Autodesk Inventor part; units mm, degrees
ref_plane "Plano inicial" through (0, 0, -25.4) normal (0, 0, 1) x (1, 0, 0)
ref_plane "Plano final" through (0, 0, 2215.4) normal (0, 0, 1) x (1, 0, 0)
ref_plane "Plano de trabajo4" through (0, 25.4, 2215.4) normal (0, -0.7071, 0.7071) x (1, 0, 0)
ref_plane "Plano inicial" through (0, 0, -25.4) normal (0, 0, 1) x (1, 0, 0)
ref_plane "Plano final" through (0, 0, 2215.4) normal (0, 0, 1) x (1, 0, 0)
sketch "Boceto" plane through (0, 0, 0) normal (0, 0, 1) x (1, 0, 0)
  line L0 (-25.4, -19.05) -> (-25.4, 19.05)
  line L1 (-19.05, 25.4) -> (19.05, 25.4)
  line L2 (25.4, 19.05) -> (25.4, -19.05)
  line L3 (19.05, -25.4) -> (-19.05, -25.4)
  arc A0 (-25.4, -19.05) -> (-19.05, -25.4) centre (-19.05, -19.05) ccw
  arc A1 (-19.05, 25.4) -> (-25.4, 19.05) centre (-19.05, 19.05) ccw
  arc A2 (25.4, 19.05) -> (19.05, 25.4) centre (19.05, 19.05) ccw
  arc A3 (19.05, -25.4) -> (25.4, -19.05) centre (19.05, -19.05) ccw
  arc A4 (-19.05, 22.225) -> (-22.225, 19.05) centre (-19.05, 19.05) ccw
  line L4 (-19.05, 22.225) -> (19.05, 22.225)
  arc A5 (22.225, 19.05) -> (19.05, 22.225) centre (19.05, 19.05) ccw
  line L5 (22.225, 19.05) -> (22.225, -19.05)
  arc A6 (19.05, -22.225) -> (22.225, -19.05) centre (19.05, -19.05) ccw
  line L6 (19.05, -22.225) -> (-19.05, -22.225)
  arc A7 (-22.225, -19.05) -> (-19.05, -22.225) centre (-19.05, -19.05) ccw
  line L7 (-22.225, -19.05) -> (-22.225, 19.05)
  line L8 (0, 37.4012) -> (0, -37.4012) construction
  line L9 (-37.4012, 0) -> (37.4012, 0) construction
  dimension "d10" = 50.8
  dimension "d11" = 50.8
  dimension "d12" = 3.175
  dimension "d15" = 25.4
  dimension "d16" = 25.4
  dimension "d17" = 6.35
extrude "Cuerpo" add sketch "Boceto" along normal up to surface (2240.8 mm away) from surface at -25.4
sketch "Sketch3" plane through (0, 0, 0) normal (0, 0, 1) x (1, 0, 0)
  line L0 (0, 0) -> (10, 0)
ref_plane "Work Plane3" through (0, 0, 0) normal (0, -1, 0) x (1, 0, 0)
ref_plane "Plano de trabajo4" through (0, 25.4, 2215.4) normal (0, -0.7071, 0.7071) x (1, 0, 0)
split "Dividir1" plane through (0, 25.4, 2215.4) removes the side toward (0, -0.7071, 0.7071)
ref_plane "Plano de trabajo5" through (0, 25.4, -25.4) normal (0, -0.7071, -0.7071) x (1, 0, 0)
split "Dividir2" plane through (0, 25.4, -25.4) removes the side toward (0, -0.7071, -0.7071)
sketch "Boceto5" plane through (-25.4, 19.05, -19.05) normal (-1, 0, 0) x (0, 0, 1)
  line L0 (19.05, -19.05) -> (2209.05, -19.05)
  line L1 (2228.1, 0) -> (2190, -38.1)
  circle A0 centre (2113.9016, -19.05) radius 9.017
  circle A1 centre (1345.45, -19.05) radius 9.017
  circle A2 centre (558.05, -19.05) radius 9.017
  line L2 (2190, -38.1) -> (2228.1, 0)
  dimension "d20" = 18.034
  dimension "d21" = 18.034
  dimension "d22" = 18.034
  dimension "d23" = 1651
  dimension "d24" = 863.6
  dimension "d25" = 95.1484
extrude "Extrusión2" cut sketch "Boceto5" against normal blind 12.7
sketch "Sketch4" plane through (0, 0, 0) normal (0, -1, 0) x (1, 0, 0)
  line L0 (-2, -25.4) -> (12, -25.4)
  line L1 (-2, 2215.4) -> (12, 2215.4)
  dimension "d19" = 2240.8
equation "\"d10\" = G_H"
equation "\"d11\" = G_W"
equation "\"d12\" = G_T"
equation "\"d15\" = 0.5 * d10"
equation "\"d16\" = 0.5 * d11"
equation "\"d17\" = G_IR"
equation "\"d3\" = G_L"
equation "\"G_W\" = 50.8"
equation "\"G_H\" = 50.8"
equation "\"G_T\" = 3.175"
equation "\"G_IR\" = 6.35"
equation "\"G_L\" = d19"
equation "\"G_OFFSET_START\" = 25.4"
equation "\"G_OFFSET_END\" = 25.4"
equation "\"d13\" = -G_OFFSET_START"
equation "\"d14\" = G_OFFSET_END + B_L"
equation "\"B_L\" = 2190"
properties part number "AISC - 2 x 2 x 1/8 - 88,22" material "Acero, suave"
Here's how the part is built. I have some questions about the finished solid (model axes, mm). A direction names the side the tool comes from. Coordinates: 2 decimals unless noted, no trailing zeros. Order: outer loops, then holes, each group sorted by start corner. A loop starts at its lowest first (then second) coordinate and runs counter-clockwise, first axis right, second up. Notation, with made-up numbers: (87.25, -12) -> (110.25, -12) arc R33 cw to (110.25, 16) -> close; hole circle Ø3 at (24, 54). An arc over 180 degrees is marked (long way). Return JSON: item names as keys, results as strings.
1) If we section it at A-A on y = 0: List the corners of the cut face in (x, z) for me (3 decimals), plus the area to 3 significant figures.
Conclusion:
{"outline": "(-25.4, 0) -> (-22.225, 0) -> (-22.225, 529.983) -> (-25.4, 529.983) -> close; (-25.4, 548.017) -> (-22.225, 548.017) -> (-22.225, 1317.383) -> (-25.4, 1317.383) -> close; (-25.4, 1335.417) -> (-22.225, 1335.417) -> (-22.225, 2085.835) -> (-25.4, 2085.835) -> close; (-25.4, 2103.869) -> (-22.225, 2103.869) -> (-22.225, 2190) -> (-25.4, 2190) -> close; (22.225, 0) -> (25.4, 0) -> (25.4, 2190) -> (22.225, 2190) -> close", "area": "13,700 mm²"}
2) If we section it at B-B on z = 1276: List the corners of the cut face in (x, y) for me (3 decimals).
Conclusion:
{"outline": "(-25.4, -19.05) arc R6.35 ccw to (-19.05, -25.4) -> (19.05, -25.4) arc R6.35 ccw to (25.4, -19.05) -> (25.4, 19.05) arc R6.35 ccw to (19.05, 25.4) -> (-19.05, 25.4) arc R6.35 ccw to (-25.4, 19.05) -> close; hole (-22.225, -19.05) arc R3.175 ccw to (-19.05, -22.225) -> (19.05, -22.225) arc R3.175 ccw to (22.225, -19.05) -> (22.225, 19.05) arc R3.175 ccw to (19.05, 22.225) -> (-19.05, 22.225) arc R3.175 ccw to (-22.225, 19.05) -> close"}
3) On a 3-axis mill with a long thin cutter (end or side, diameter ignored), from which of +Z, -Z, +X, -X, +Y, -Y can I reach the whole of each face in a straight line? I mean faces 1 (the flat face through (-22.225, 0, 1079)), 2 (the flat face through (22.5, -0.1, 2189.9)). Say none if no direction works.
Conclusion:
{"face 1": "+Z, -Z", "face 2": "+Z, +X, -X, -Y"}
4) I'm going to push flat-ended pins straight in: P1, Ø14.5, axis at y = 0, z = 539, coming from the -X side (3 decimals); P2, Ø12, axis at x = -19, y = 10.5, coming from the -Z side; P3, Ø10, axis at x = -18.5, y = 13, coming from the -Z side. Where does each tip first touch, or does it pass through?
Conclusion:
{"P1": "stops at x = 22.225", "P2": "stops at z = -15.56", "P3": "stops at z = -16.34"}
5) If I drill on probe 1 along X at (y, z) = (13.5, 1417.5) (3 decimals); probe 2 along Z at (x, y) = (-24.7, 0), over which ranges is the centre line in solid material (lowest first)?
Conclusion:
{"probe 1": "x = -25.4 to -22.225, 22.225 to 25.4", "probe 2": "z = 0 to 529.98, 548.02 to 1317.38, 1335.42 to 2085.83, 2103.87 to 2190"}
6) Thinking about a two-plate mould opening in X: for faces 3 (the flat face through (22.5, 0.1, -0.1)), 4 (the flat face through (0, -22.225, 1080)), 5 (the flat face through (-25.4, 0, 1079)), which applies, +X half, -X half, draft (parallel to the pull), parting line (faces both ways), or undercut?
Conclusion:
{"face 3": "draft", "face 4": "undercut", "face 5": "-X half"}
